Source: CAD feature listing. Evaluate the final solid. Frame: model axes, mm. Give positions to 0.01 mm unless a question says otherwise; leave off trailing zeros. Order: outer loops, then holes, each group sorted by start corner. A loop starts at its lowest first (then second) coordinate and runs counter-clockwise, first axis right, second up.
1) Material intervals for line 1 (Y direction, x = -2.25, z = 28.5); line 2 (Y direction, x = 0.5, z = 133); line 3 (X direction, y = -3.25, z = 19.5), sorted ascending.
2) Section A-A, the plane z = -54. Return loops of the section in (x, y).
3) First-contact query: P1, Ø3, axis at y = -3.5, z = -46.5, coming from the -X side; P2, Ø5, axis at x = -2.5, z = 65.5, coming from the -Y side; P3, Ø1, axis at y = 2, z = -34, coming from the +X side; P4, Ø1.5, axis at y = 2, z = -158, coming from the -X side. Flat tips, straight axial feed; report the tip coordinate or a pass-through.
```python
from build123d import *

# Parameters (mm, degrees)
SKETCH3_R                = 5
BOSS_EXTRUDE2_DEPTH      = 200
BOSS_EXTRUDE2_DEPTH_BACK = 200
CUT_EXTRUDE5_DEPTH       = 201
CUT_EXTRUDE5_DEPTH_BACK  = 201
CHAMFER1_SIZE            = 0.5


with BuildPart() as part:
    # Sketch3 → Boss-Extrude2 (new body, two sides)
    with BuildSketch(Plane.XY) as boss_extrude2_sk:
        Circle(SKETCH3_R)
    extrude(amount=BOSS_EXTRUDE2_DEPTH)
    extrude(boss_extrude2_sk.sketch, amount=-BOSS_EXTRUDE2_DEPTH_BACK)

    # Sketch10 → Cut-Extrude5 (cut, two sides)
    with BuildSketch(Plane.XY) as cut_extrude5_sk:
        with BuildLine():
            Line((-2.5, 4.330127019), (2.5, 4.330127019))
            ThreePointArc((2.5, 4.330127019), (0, 5), (-2.5, 4.330127019))
        make_face()
    extrude(amount=CUT_EXTRUDE5_DEPTH, mode=Mode.SUBTRACT)
    extrude(cut_extrude5_sk.sketch, amount=-CUT_EXTRUDE5_DEPTH_BACK, mode=Mode.SUBTRACT)

    # Chamfer1
    chamfer1_edges = [part.edges().sort_by_distance(p)[0] for p in [
        (0, -5, -200),
        (0, -5, 200),
    ]]
    chamfer(chamfer1_edges, length=CHAMFER1_SIZE)


solid = part.part
```
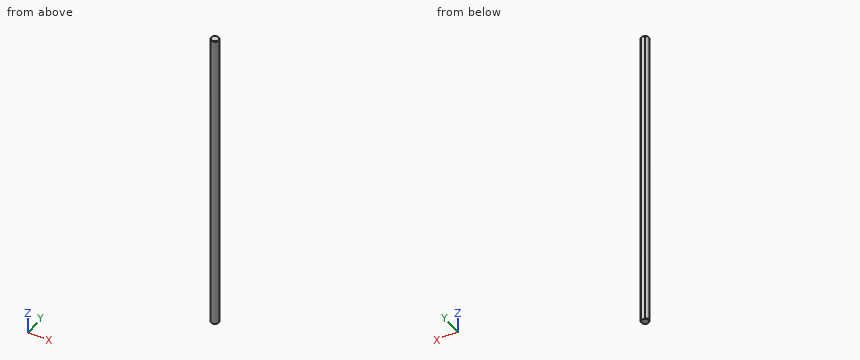
From the geometry:
1. line 1: y = -4.47 to 4.33
1. line 2: y = -4.97 to 4.33
1. line 3: x = -3.8 to 3.8
2. outline: (-2.5, 4.33) arc R5 ccw (long way) to (2.5, 4.33) - close
3. P1: stops at x = -4.58
3. P2: stops at y = -5
3. P3: stops at x = 4.77
3. P4: stops at x = -4.84
